Could you check a few things on this model? Use its own coordinates, in mm. Face numbers are marked on the shaded views. A direction names the side the tool comes from. Coordinates: 2 decimals unless noted, no trailing zeros. Loops run counter-clockwise (first coordinate to the right, second up) from the corner with the lowest first, then second, coordinate; pieces in that order, holes last.
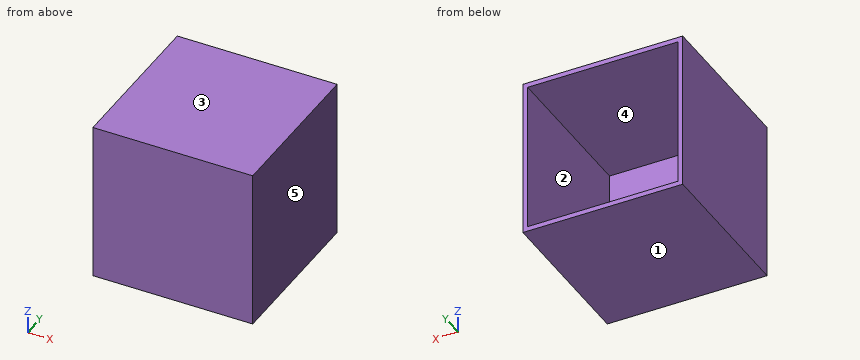
from build123d import *

# Parameters (mm, degrees)
SKETCH1_W           = 1000
SKETCH1_H           = 1000
BOSS_EXTRUDE1_DEPTH = 1000
SHELL1_T            = -30
SKETCH4_W           = 140
SKETCH4_H           = 140
BOSS_EXTRUDE2_DEPTH = 200
SKETCH5_W           = 60
SKETCH5_H           = 50
BOSS_EXTRUDE3_DEPTH = 20
SKETCH6_R           = 10
CUT_EXTRUDE5_DEPTH  = 80


with BuildPart() as part:
    # Sketch1 → Boss-Extrude1 (new body)
    with BuildSketch(Plane(origin=(0, 0, 0), x_dir=(1, 0, 0), z_dir=(0, 1, 0))):
        with Locations((410.346861064, 441.605744818)):
            Rectangle(SKETCH1_W, SKETCH1_H)
    extrude(amount=BOSS_EXTRUDE1_DEPTH)

    # Shell1
    shell1_openings = [part.faces().sort_by_distance(p)[0] for p in [
        (410.346861064, 1000, -441.605744818),
    ]]
    offset(amount=SHELL1_T, openings=shell1_openings, kind=Kind.INTERSECTION)

    # Sketch4 → Boss-Extrude2 (add)
    with BuildSketch(Plane(origin=(0, 30, 0), x_dir=(1, 0, 0), z_dir=(0, 1, 0))):
        with Locations((410.346861064, 441.605744818)):
            Rectangle(SKETCH4_W, SKETCH4_H)
    extrude(amount=BOSS_EXTRUDE2_DEPTH)

    # Sketch5 → Boss-Extrude3 (add)
    with BuildSketch(Plane(origin=(480.346861064, 0, 0), x_dir=(0, 0, -1), z_dir=(1, 0, 0))):
        with Locations((401.605744818, 55)):
            Rectangle(SKETCH5_W, SKETCH5_H)
    extrude(amount=BOSS_EXTRUDE3_DEPTH)

    # Sketch6 → Cut-Extrude5 (cut)
    with BuildSketch(Plane(origin=(0, 230, 0), x_dir=(1, 0, 0), z_dir=(0, 1, 0))):
        with Locations((410.346861064, 491.605744818)):
            Circle(SKETCH6_R)
        with Locations((360.346861064, 441.605744818)):
            Circle(SKETCH6_R)
        with Locations((410.346861064, 391.605744818)):
            Circle(SKETCH6_R)
        with Locations((460.346861064, 441.605744818)):
            Circle(SKETCH6_R)
    extrude(amount=-CUT_EXTRUDE5_DEPTH, mode=Mode.SUBTRACT)


solid = part.part
(1) Imagine slicing it at B-B, the plane x = 294. Write out the boundary of the cut face in (y, z), and give its area (3 significant figures).
Answers:
outline: (0, -941.61) - (1000, -941.61) - (1000, -911.61) - (30, -911.61) - (30, 28.39) - (1000, 28.39) - (1000, 58.39) - (0, 58.39) - close
area: 88,200 mm2
(2) I need wall thicknesses on probe 1 along Z at (x, y) = (209.5, 394); probe 2 along X at (y, z) = (187, -713); probe 3 along Y at (x, z) = (281, -346.5). Which ranges of each line are inside material? Lowest first, please.
Answers:
probe 1: z = -941.61 to -911.61, 28.39 to 58.39
probe 2: x = -89.65 to -59.65, 880.35 to 910.35
probe 3: y = 0 to 30
(3) For pin 1 (1.5 mm diameter, centred on x = 291, z = -221, fed in from +Y); pin 2 (6 mm diameter, centred on x = 408.5, z = -392, fed in from +Y); pin 3 (22 mm diameter, centred on x = 409.5, z = -489.5, fed in from +Y), each with a flat end and sliding along its axis, tell me the tip position at first contact or that it passes through.
Answers:
pin 1: stops at y = 30
pin 2: stops at y = 150
pin 3: stops at y = 230
(4) Imagine slicing it at C-C, the plane y = 889.5. Write out the boundary of the cut face in (x, z).
Answers:
outline: (-89.65, -941.61) - (910.35, -941.61) - (910.35, 58.39) - (-89.65, 58.39) - close; hole (-59.65, -911.61) - (880.35, -911.61) - (880.35, 28.39) - (-59.65, 28.39) - close
(5) Which directions (+Z, -Z, +X, -X, +Y, -Y) give clear straight access to the entire face, cutting with the end or side of a thin tool? Please do the marked faces 1 and 2.
Answers:
face 1: -Z, +X, -X, +Y, -Y
face 2: +Y
(6) We'd pull the mould along X, two halves only. Please class the marked faces 3, 4 and 5: +X half, -X half, draft (parallel to the pull), parting line (faces both ways), or undercut.
Answers:
face 3: draft
face 4: undercut
face 5: +X half
(7) Imagine slicing it at D-D, the plane z = -853. Write out the boundary of the cut face in (x, y).
Answers:
outline: (-89.65, 0) - (910.35, 0) - (910.35, 1000) - (880.35, 1000) - (880.35, 30) - (-59.65, 30) - (-59.65, 1000) - (-89.65, 1000) - close
(8) Imagine slicing it at A-A, the plane y = 99.5. Write out the boundary of the cut face in (x, z).
Answers:
outline: (-89.65, -941.61) - (910.35, -941.61) - (910.35, 58.39) - (-89.65, 58.39) - close; (340.35, -511.61) - (480.35, -511.61) - (480.35, -371.61) - (340.35, -371.61) - close; hole (-59.65, -911.61) - (880.35, -911.61) - (880.35, 28.39) - (-59.65, 28.39) - close
